```python
from build123d import *

# Parameters (mm, degrees)
SKETCH1_R      = 3.9624
EXTRUDE1_DEPTH = 2.2098
FILLET1_R      = 1.524
SKETCH2_R      = 2.0828
EXTRUDE2_DEPTH = 25.4
EXTRUDE3_DEPTH = 1.016


with BuildPart() as part:
    # Sketch1 → Extrude1 (new body)
    with BuildSketch(Plane.XY):
        Circle(SKETCH1_R)
    extrude(amount=EXTRUDE1_DEPTH)

    # Fillet1
    fillet1_edges = [part.edges().sort_by_distance(p)[0] for p in [
        (-3.9624, 0, 0),
    ]]
    fillet(fillet1_edges, radius=FILLET1_R)

    # Sketch2 → Extrude2 (add)
    with BuildSketch(Plane.XY.offset(2.2098)):
        Circle(SKETCH2_R)
    extrude(amount=EXTRUDE2_DEPTH)

    # Sketch3 → Extrude3 (cut)
    with BuildSketch(Plane(origin=(0, 0, 0), x_dir=(-1, 0, 0), z_dir=(0, 0, -1))):
        Polygon((0.709024608, 1.177879999), (-0.665561698, 1.202973322), (-1.374586306, 0.025093323), (-0.709024608, -1.177879999), (0.665561698, -1.202973322), (1.374586306, -0.025093323), align=None)
    extrude(amount=-EXTRUDE3_DEPTH, mode=Mode.SUBTRACT)


solid = part.part
```
Source: CAD feature listing. Evaluate the final solid. Frame: model axes, mm. A direction names the side the tool comes from. Give positions to 0.01 mm unless a question says otherwise; leave off trailing zeros. Write each loop counter-clockwise with the first axis right and the second up, starting at its lowest first coordinate (ties: lowest second). Pieces come first, ordered by that corner, then holes. Notation, with made-up numbers: (36, 75) - (58, 75) arc R20 ccw to (58, 92) - close; hole circle Ø7 at (-26.5, 33). An arc over 180 degrees is marked (long way). One line per item, written item: value. Start each with the question number.
Q1. Material intervals for probe 1 along Z at (x, y) = (-0.25, -0.5); probe 2 along Z at (x, y) = (-1.5, -2); probe 3 along Y at (x, z) = (0, 15.25), sorted ascending. Write a range as from..to.
Q2. First-contact query: pin 1 Ø1.5 at (y, z) = (-1.5, 24.5) entering from +X; pin 2 Ø1 at (x, z) = (-1, 6.5) entering from +Y; pin 3 Ø4 at (y, z) = (0.5, 16.5) entering from +X. Flat tips, straight axial feed; report the tip coordinate or a pass-through.
Q3. Draft query along Y for faces 1 (the face through (0, 0, 1.016)), 2 (the face through (1.987, 0.626, 14.732)), 3 (the face through (0, 0, 27.61)). Return one class per face: +Y half, -Y half, draft (parallel to the pull), parting line (faces both ways), or undercut.
Q4. Section query B-B, the plane z = 25.25. Return the cut outline in (x, y).
Q5. Section query A-A, the plane x = 0. Return the cut outline in (y, z), then the cut area to 3 significant figures.
Q6. Set-up query: faces 4 (the face through (1.046, -0.568, 0.501)), 5 (the face through (-0.52, 3.93, 1.86)), 6 (the face through (2, -2, 2.21)). Return all of +Z, -Z, +X, -X, +Y, -Y with unobstructed straight access to the full face (end or side cutting, diameter ignored); none if empty.
Answer:
1. probe 1: z = 1.02..27.61
1. probe 2: z = 0..2.21
1. probe 3: y = -2.08..2.08
2. pin 1: stops at x = 1.94
2. pin 2: stops at y = 2.02
2. pin 3: stops at x = 2.08
3. face 1: undercut
3. face 2: parting line
3. face 3: draft
4. outline: circle Ø4.17 at (0, 0)
5. outline: (-3.96, 1.52) arc R1.52 ccw to (-2.44, 0) - (-1.19, 0) - (-1.19, 1.02) - (1.19, 1.02) - (1.19, 0) - (2.44, 0) arc R1.52 ccw to (3.96, 1.52) - (3.96, 2.21) - (2.08, 2.21) - (2.08, 27.61) - (-2.08, 27.61) - (-2.08, 2.21) - (-3.96, 2.21) - close
5. area: 120 mm2
6. face 4: -Z
6. face 5: +Z, -Z
6. face 6: +Z
